Verification items for the finished model (mm, model axes). Round coordinates to 2 decimals unless told otherwise and drop trailing zeros. Order: outer loops, then holes, each group sorted by start corner. A loop starts at its lowest first (then second) coordinate and runs counter-clockwise, first axis right, second up. Notation, with made-up numbers: M 81,50 L 87,50 A16 ccw 87,74 Z; hole C -28.5,48.25 d7. An arc over 180 degrees is marked long. Return JSON: item names as keys, results as strings. Group by question number.
from build123d import *

# Parameters (mm, degrees)
SZKIC1_W                    = 1300
SZKIC1_H                    = 496.747706102
DODANIE_WYCI_GNI_CIE1_DEPTH = 50
WYTNIJ_WYCI_GNI_CIE1_DEPTH  = 30
SZKIC3_W                    = 200.09890069
SZKIC3_H                    = 50
DODANIE_WYCI_GNI_CIE2_DEPTH = 497


with BuildPart() as part:
    # Szkic1 → Dodanie-wyciągnięcie1 (new body)
    with BuildSketch(Plane.XY):
        with Locations((-650, 248.373853051)):
            Rectangle(SZKIC1_W, SZKIC1_H)
    extrude(amount=DODANIE_WYCI_GNI_CIE1_DEPTH)

    # Szkic2 → Wytnij-wyciągnięcie1 (cut)
    with BuildSketch(Plane.XY.offset(60)):
        Polygon((-978.316280033, 248.373853051), (-978.316280033, 343.566812888), (-938.316280033, 343.566812888), (-938.316280033, 128.566812888), (-978.316280033, 128.566812888), align=None)
        Polygon((-667.389420711, 248.373853051), (-667.389420711, 343.566812888), (-627.389420711, 343.566812888), (-627.389420711, 128.566812888), (-667.389420711, 128.566812888), align=None)
    extrude(amount=-WYTNIJ_WYCI_GNI_CIE1_DEPTH, mode=Mode.SUBTRACT)

    # Szkic3 → Dodanie-wyciągnięcie2 (add)
    with BuildSketch(Plane(origin=(0, 0, 0), x_dir=(-1, 0, 0), z_dir=(0, -1, 0))):
        with Locations((1400.049450345, -25)):
            Rectangle(SZKIC3_W, SZKIC3_H)
    extrude(amount=-DODANIE_WYCI_GNI_CIE2_DEPTH)


solid = part.part
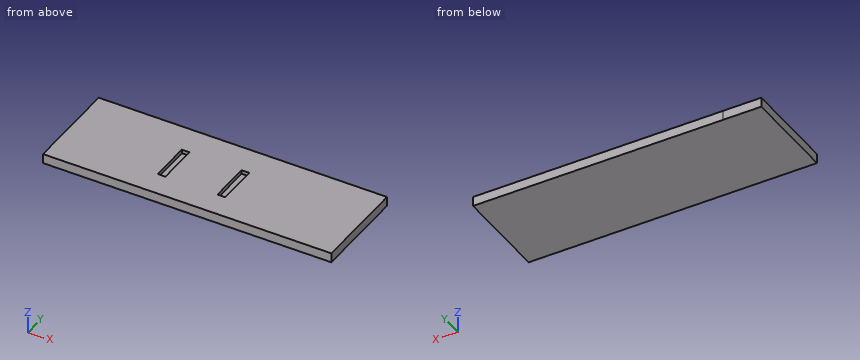
1. Thickness scan on line 1 along X through (y, z) = (211.5, 45.5); line 2 along Y through (x, z) = (-399.5, 22.5). Record the ranges inside material, lowest first. Write a range as from..to.
2. Go/stop test with a flat-tipped pin: pin 1 (15 mm diameter, centred on x = -476, z = 25, fed in from +Y). Record where the tip stops, or that it passes through.
3. Cross-section at A-A (z = 39). Enter the section's corners in (x, y).
4. Cross-section at B-B (y = 296). Enter the section's corners in (x, z), plus the area to 3 significant figures.
Computed:
{
 "1": {"line 1": "x = -1500.1..-978.32, -938.32..-667.39, -627.39..0", "line 2": "y = 0..496.75"},
 "2": {"pin 1": "stops at y = 496.75"},
 "3": {"outline": "M -1500.1,0 L 0,0 L 0,496.75 L -1300,496.75 L -1300,497 L -1500.1,497 Z; hole M -978.32,128.57 L -938.32,128.57 L -938.32,343.57 L -978.32,343.57 Z; hole M -667.39,128.57 L -627.39,128.57 L -627.39,343.57 L -667.39,343.57 Z"},
 "4": {"outline": "M -1500.1,0 L 0,0 L 0,50 L -627.39,50 L -627.39,30 L -667.39,30 L -667.39,50 L -938.32,50 L -938.32,30 L -978.32,30 L -978.32,50 L -1500.1,50 Z", "area": "73,400 mm²"}
}
